from build123d import *

# Parameters (mm, degrees)
F0_W     = 43
F0_H     = 3
F1_DEPTH = 25


with BuildPart() as f1:
    # F0 (on Top) → F1 (new body)
    with BuildSketch(Plane.XY):
        with Locations((9.041131, 14.730754)):
            Rectangle(F0_W, F0_H)
        Polygon((-12.458869, 13.230754), (-12.458869, 16.230754), (-15.458869, 16.230754), (-15.458869, -13.769246), (-12.458869, -13.769246), align=None)
        Polygon((33.541131, 16.230754), (30.541131, 16.230754), (30.541131, 13.230754), (30.541131, -13.769246), (33.541131, -13.769246), align=None)
    extrude(amount=F1_DEPTH)


solid = f1.part
Source: CAD feature listing. Evaluate the final solid. Frame: model axes, mm. A direction names the side the tool comes from. Give positions to 0.01 mm unless a question says otherwise; leave off trailing zeros. Order: outer loops, then holes, each group sorted by start corner. A loop starts at its lowest first (then second) coordinate and runs counter-clockwise, first axis right, second up. Notation, with made-up numbers: (15, 7) -> (32, 7) arc R28 ccw to (32, 39) -> close; hole circle Ø4 at (50.25, 40). An arc over 180 degrees is marked (long way). Write item = value, one per line.
Item 1: Contact query for a flat-ended pin moving along its axis: pin 1 (12.5 mm diameter, centred on x = -1, z = 11.5, fed in from -Y). Output: stop coordinate, or through.
Check result:
pin_1 = 13.23
Item 2: Mould query, pull axis X, two halves, no side actions, for faces 3 (the face through (-12.459, 0, 12)), 4 (the face through (9, 14, 25)), 5 (the face through (-15.459, 1, 12)). Classes: +X half, -X half, draft (parallel to the pull), parting line (faces both ways), or undercut.
Check result:
face_3 = undercut
face_4 = draft
face_5 = -X half
Item 3: Set-up query: faces 1 (the face through (9, 13.231, 12)), 2 (the face through (9, 14, 0)). Return all of +Z, -Z, +X, -X, +Y, -Y with unobstructed straight access to the full face (end or side cutting, diameter ignored); none if empty.
Check result:
face_1 = +Z, -Z, -Y
face_2 = -Z, +X, -X, +Y, -Y
Item 4: Section query C-C (x = 16). Output: boundary loops of the cut face in (y, z).
Check result:
outline = (13.23, 0) -> (16.23, 0) -> (16.23, 25) -> (13.23, 25) -> close
Item 5: Section query A-A (y = 1.5). Output: boundary loops of the cut face in (x, z), then the cut area to 3 significant figures.
Check result:
outline = (-15.46, 0) -> (-12.46, 0) -> (-12.46, 25) -> (-15.46, 25) -> close; (30.54, 0) -> (33.54, 0) -> (33.54, 25) -> (30.54, 25) -> close
area = 150 mm²
Item 6: Section query B-B (z = 15). Output: boundary loops of the cut face in (x, y).
Check result:
outline = (-15.46, -13.77) -> (-12.46, -13.77) -> (-12.46, 13.23) -> (30.54, 13.23) -> (30.54, -13.77) -> (33.54, -13.77) -> (33.54, 16.23) -> (-15.46, 16.23) -> close
Item 7: Ray query, probe 1 along X at (y, z) = (-4.25, 17.5); probe 2 along Y at (x, z) = (11, 22). Return the intervals inside material, ascending.
Check result:
probe_1 = -15.46 to -12.46, 30.54 to 33.54
probe_2 = 13.23 to 16.23
